from build123d import *

# Parameters (mm, degrees)
SKETCH_1_W      = 36
SKETCH_1_H      = 36
EXTRUDE_1_DEPTH = 10
SKETCH_3_R      = 8
EXTRUDE_2_DEPTH = 25
SKETCH_4_W      = 27
SKETCH_4_H      = 3.9
EXTRUDE_3_DEPTH = 2.063094661
SKETCH_5_W      = 27
SKETCH_5_H      = 3.9
EXTRUDE_4_DEPTH = 2.063094661
SKETCH_6_R      = 2.5
EXTRUDE_5_DEPTH = 2.063094661


with BuildPart() as part:
    # 草图1 → 凸台-拉伸1 (new body)
    with BuildSketch(Plane(origin=(0, 0, 0), x_dir=(1, 0, 0), z_dir=(0, 1, 0))):
        Rectangle(SKETCH_1_W, SKETCH_1_H)
    extrude(amount=EXTRUDE_1_DEPTH)

    # 草图3 → 凸台-拉伸2 (add)
    with BuildSketch(Plane(origin=(0, 10, 0), x_dir=(1, 0, 0), z_dir=(0, 1, 0))):
        with Locations(Location((0, 5, 0), (0, 0, 270))):
            Circle(SKETCH_3_R)
    extrude(amount=EXTRUDE_2_DEPTH)

    # 草图4 → 凸台-拉伸3 (add)
    with BuildSketch(Plane.ZY.offset(18)):
        with Locations((13.5, 5)):
            Rectangle(SKETCH_4_W, SKETCH_4_H)
    extrude(amount=EXTRUDE_3_DEPTH)

    # 草图5 → 凸台-拉伸4 (add)
    with BuildSketch(Plane(origin=(18, 0, 0), x_dir=(0, 0, -1), z_dir=(1, 0, 0))):
        with Locations((-13.5, 5)):
            Rectangle(SKETCH_5_W, SKETCH_5_H)
    extrude(amount=EXTRUDE_4_DEPTH)

    # 草图6 → 凸台-拉伸5 (add)
    with BuildSketch(Plane.XY.offset(27)):
        with BuildLine():
            Line((20.063094661, 3.05), (20.063094661, 0))
            Line((20.063094661, 0), (8.660254038, 0))
            ThreePointArc((8.660254038, 0), (0, -5), (-8.660254038, 0))
            Line((-8.660254038, 0), (-20.063094661, 0))
            Line((-20.063094661, 0), (-20.063094661, 10))
            Line((-20.063094661, 10), (-8.660254038, 10))
            ThreePointArc((-8.660254038, 10), (0, 15), (8.660254038, 10))
            Line((8.660254038, 10), (20.063094661, 10))
            Line((20.063094661, 10), (20.063094661, 3.05))
        make_face()
        with Locations((0, 5)):
            Circle(SKETCH_6_R, mode=Mode.SUBTRACT)
    extrude(amount=EXTRUDE_5_DEPTH)


solid = part.part
Geometry: final body of the model. Coordinates: model frame, mm. A direction names the side the tool comes from. Coordinates: 2 decimals unless noted, no trailing zeros. Loops run counter-clockwise (first coordinate to the right, second up) from the corner with the lowest first, then second, coordinate; pieces in that order, holes last. Notation, with made-up numbers: (60, -22.5) - (73, -22.5) arc R3 ccw to (73, -17.5) - close; hole circle Ø7 at (15, -15). An arc over 180 degrees is marked (long way). Put each result on its own line as item: value. Start each with the question number.
Q1. Cut plane D-D, the plane y = 5. Return loops of the section in (x, z).
Q2. Pull-direction query (X, two-part tool) for faces 4 (the flat face through (-20.063, 5, 18)), 5 (the cylindrical face through (-4.868, 22.325, -11.349)), 6 (the flat face through (-18, 5, 22)); classes: released by +X, released by -X, zero draft, split by the parting line, or undercut.
Q3. Cut plane B-B, the plane y = 1. Return loops of the section in (x, z), and give its area (3 significant figures).
Q4. Pin query (flat end, axial travel): pin 1 Ø0.6 at (x, z) = (-13, 28) entering from -Y; pin 2 Ø1 at (x, z) = (19, 16) entering from +Y; pin 3 Ø8 at (y, z) = (7.5, -7) entering from +X; pin 4 Ø10 at (y, z) = (19.5, 11) entering from -X. Return the tip coordinate at first contact, or that it passes through.
Q5. Line query: line 1 (Z direction, x = 12.5, y = 5.5); line 2 (X direction, y = 2.5, z = 4.5); line 3 (Y direction, x = -6, z = 0). Output: solid intervals per line, ascending.
Q6. Cut plane A-A, the plane x = -12. Return loops of the section in (y, z), and give its area (3 significant figures).
Q7. Cut plane C-C, the plane z = -5. Return loops of the section in (x, y).
Q8. Set-up query: faces 1 (the flat face through (0, 10, 4)), 2 (the flat face through (19, 6.95, 14)), 3 (the flat face through (-14, 10, 28)). Return all of +Z, -Z, +X, -X, +Y, -Y with unobstructed straight access to the full face (end or side cutting, diameter ignored); none if empty.
Filled sheet:
1. outline: (-20.06, 0) - (-18, 0) - (-18, -18) - (18, -18) - (18, 0) - (20.06, 0) - (20.06, 29.06) - (2.5, 29.06) - (2.5, 27) - (18, 27) - (18, 18) - (-18, 18) - (-18, 27) - (-2.5, 27) - (-2.5, 29.06) - (-20.06, 29.06) - close
2. face 4: released by -X
2. face 5: split by the parting line
2. face 6: undercut
3. outline: (-20.06, 27) - (20.06, 27) - (20.06, 29.06) - (-20.06, 29.06) - close; (-18, -18) - (18, -18) - (18, 18) - (-18, 18) - close
3. area: 1,380 mm²
4. pin 1: y = 0
4. pin 2: y = 6.95
4. pin 3: x = 18
4. pin 4: through
5. line 1: -18 to 18, 27 to 29.06
5. line 2: -18 to 18
5. line 3: 0 to 35
6. outline: (0, -18) - (10, -18) - (10, 18) - (0, 18) - close; (0, 27) - (10, 27) - (10, 29.06) - (0, 29.06) - close
6. area: 381 mm²
7. outline: (-18, 0) - (18, 0) - (18, 10) - (8, 10) - (8, 35) - (-8, 35) - (-8, 10) - (-18, 10) - close
8. face 1: +Y
8. face 2: -Z, +X, +Y
8. face 3: +Z, -Z, -X, +Y
